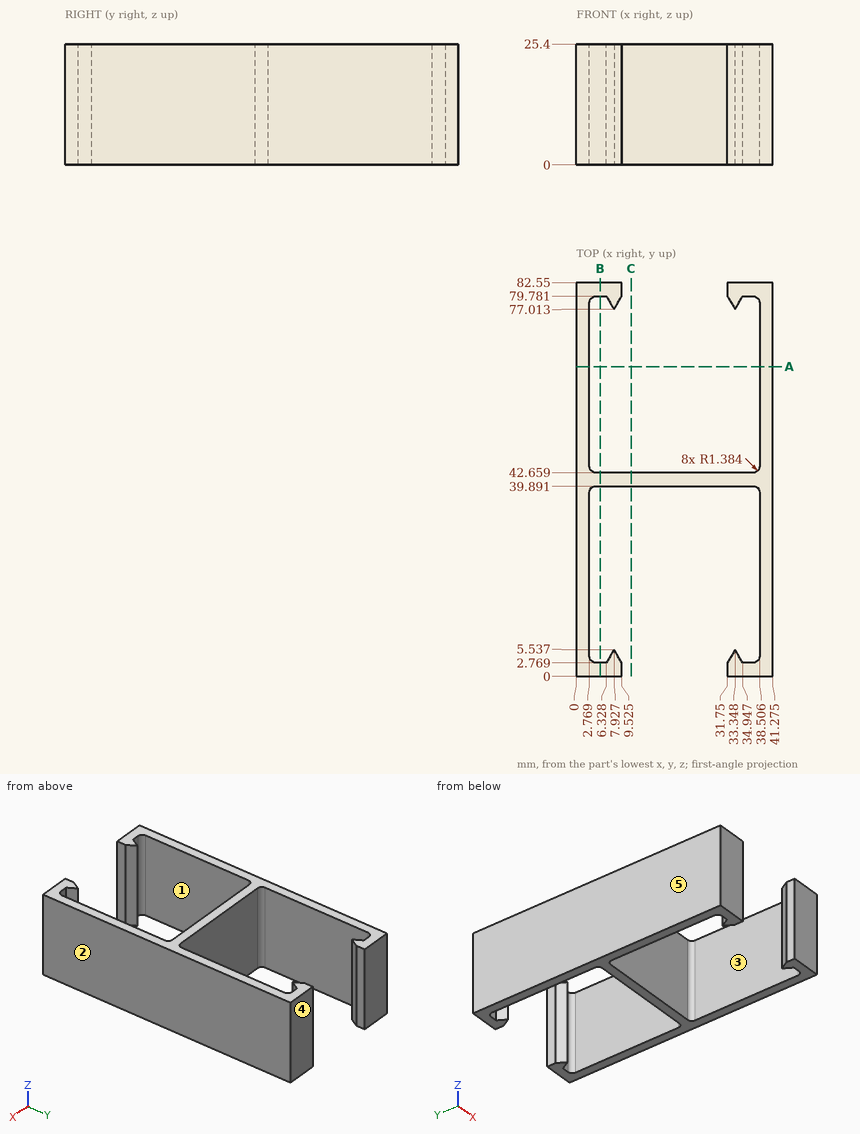
For this review, use the dimensioned drawing (mm, ordinates from the lowest corner) and the shaded views. A direction names the side the tool comes from. Give positions to 0.01 mm unless a question says otherwise; leave off trailing zeros. Loops run counter-clockwise (first coordinate to the right, second up) from the corner with the lowest first, then second, coordinate; pieces in that order, holes last.
Item 1: For line 1 along Y through (x, z) = (36, 11); line 2 along X through (y, z) = (24.5, 1.5) (1 decimal); line 3 along X through (y, z) = (79, 3.25) (1 decimal), list the stretches that pass through material, from the lowest coordinate up.
Item 2: Draft analysis for pull direction X (two halves, no side actions). For the marked faces 3, 4 and 5, state which applies: +X half, -X half, draft (parallel to the pull), parting line (faces both ways), or undercut.
Item 3: Tool access review of the marked faces 1 and 2: name each direction out of +Z, -Z, +X, -X, +Y, -Y from which nothing blocks a thin tool from reaching the whole face with its end or side.
Item 4: Take a section at B-B, the plane x = 5. State the section outline as (y, z) points.
Item 5: Take a section at C-C, the plane x = 11.5. State the section outline as (y, z) points.
Item 6: Insertion check: pin 1 (4 mm diameter, centred on x = 20, z = 2.5, fed in from -Y); pin 2 (12.5 mm diameter, centred on x = 19.5, z = 9, fed in from +Y). Each pin has a flat end and moves straight along its axis. Give the tip position at first contact, or say it passes through.
Item 7: Take a section at A-A, the plane y = 65. State the section outline as (x, z) points (1 decimal), and give its area (3 significant figures).
Calculated:
1. line 1: y = 0 to 2.77, 39.89 to 42.66, 79.78 to 82.55
1. line 2: x = 0 to 2.8, 38.5 to 41.3
1. line 3: x = 0 to 2.9, 6.8 to 9.1, 32.2 to 34.5, 38.4 to 41.3
2. face 3: undercut
2. face 4: draft
2. face 5: -X half
3. face 1: +Z, -Z
3. face 2: +Z, -Z, +X, +Y, -Y
4. outline: (0, 0) - (2.77, 0) - (2.77, 25.4) - (0, 25.4) - close; (39.89, 0) - (42.66, 0) - (42.66, 25.4) - (39.89, 25.4) - close; (79.78, 0) - (82.55, 0) - (82.55, 25.4) - (79.78, 25.4) - close
5. outline: (39.89, 0) - (42.66, 0) - (42.66, 25.4) - (39.89, 25.4) - close
6. pin 1: stops at y = 39.89
6. pin 2: stops at y = 42.66
7. outline: (0, 0) - (2.8, 0) - (2.8, 25.4) - (0, 25.4) - close; (38.5, 0) - (41.3, 0) - (41.3, 25.4) - (38.5, 25.4) - close
7. area: 141 mm2
